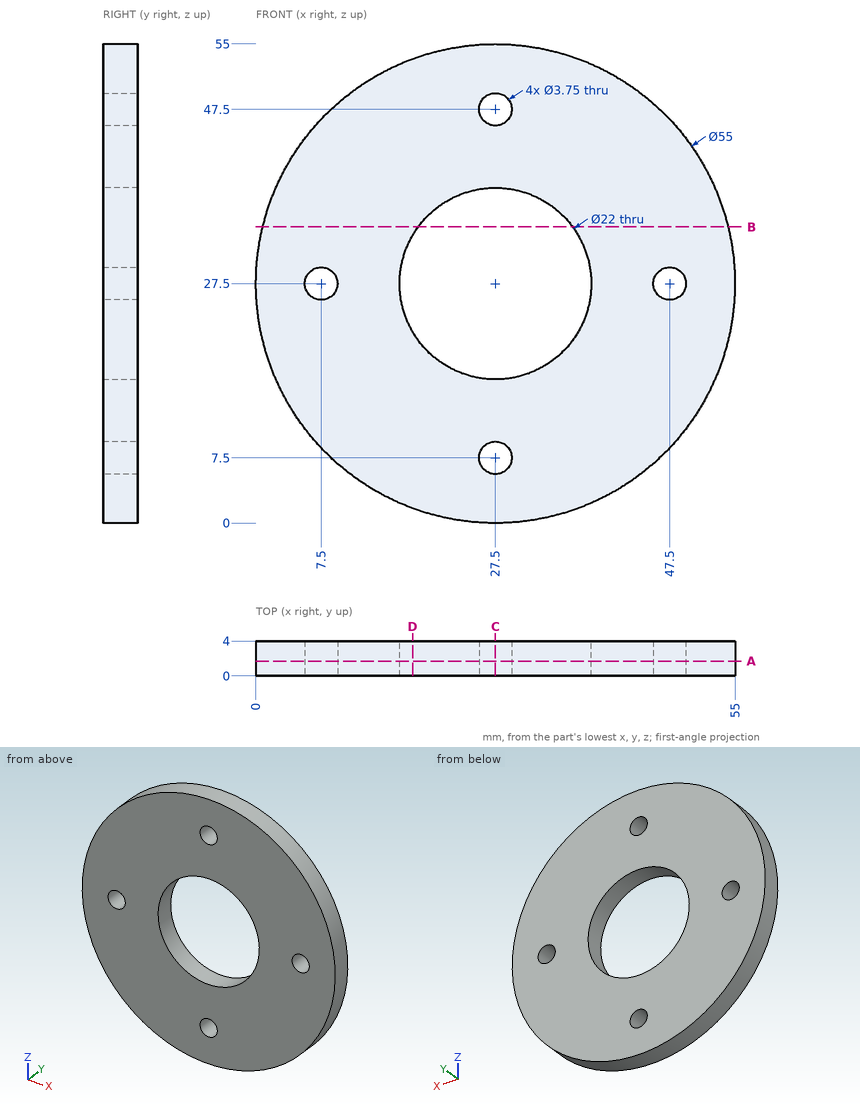
Design review of the part shown in the three views and the two pictorial views. Dimensions are in mm from the part's minimum x, y and z. Give positions to 0.01 mm unless a question says otherwise; leave off trailing zeros. Write each loop counter-clockwise with the first axis right and the second up, starting at its lowest first coordinate (ties: lowest second). Pieces come first, ordered by that corner, then holes. Notation, with made-up numbers: M -18,-11.5 L 20,-11.5 A27 cw 20,19.5 Z; hole C -9.5,40 d1. An arc over 180 degrees is marked long. Answer in a Markdown table with one row per item.
Item 1: For line 1 along X through (y, z) = (2.25, 27.5) (3 decimals); line 2 along X through (y, z) = (0.2, 28.5); line 3 along Z through (x, y) = (28, 1), list the stretches that pass through material, from the lowest coordinate up.
Check sheet entries:
| item | result |
|---|---|
| line 1 | 0 to 5.625, 9.375 to 16.5, 38.5 to 45.625, 49.375 to 55 |
| line 2 | 0.02 to 5.91, 9.09 to 16.55, 38.45 to 45.91, 49.09 to 54.98 |
| line 3 | 0 to 5.69, 9.31 to 16.51, 38.49 to 45.69, 49.31 to 55 |
Item 2: Add section A-A on y = 1.7. Give the boundary of the cut face in (x, z) (3 decimals).
Check sheet entries:
| item | result |
|---|---|
| outline | C 27.5,27.5 d55; hole C 7.5,27.5 d3.75; hole C 27.5,27.5 d22; hole C 27.5,7.5 d3.75; hole C 27.5,47.5 d3.75; hole C 47.5,27.5 d3.75 |
Item 3: Add section D-D on x = 18. Give the boundary of the cut face in (y, z).
Check sheet entries:
| item | result |
|---|---|
| outline | M 0,1.69 L 4,1.69 L 4,21.95 L 0,21.95 Z; M 0,33.05 L 4,33.05 L 4,53.31 L 0,53.31 Z |
Item 4: For P1, Ø1, axis at x = 9.5, y = 3.5, coming from the -Z side; P2, Ø1.5, axis at y = 3, z = 38.5, coming from the -X side; P3, Ø2, axis at y = 2, z = 18.5, coming from the +X side, all flat-tipped, find the tip position at first contact; note any pin that passes through.
Check sheet entries:
| item | result |
|---|---|
| P1 | z = 6.29 |
| P2 | x = 1.98 |
| P3 | x = 53.81 |
Item 5: Add section B-B on z = 34. Give the boundary of the cut face in (x, y), plus the area to 3 significant figures.
Check sheet entries:
| item | result |
|---|---|
| outline | M 0.78,0 L 18.63,0 L 18.63,4 L 0.78,4 Z; M 36.37,0 L 54.22,0 L 54.22,4 L 36.37,4 Z |
| area | 143 mm2 |
Item 6: Add section C-C on x = 27.5. Give the boundary of the cut face in (y, z) (3 decimals).
Check sheet entries:
| item | result |
|---|---|
| outline | M 0,0 L 4,0 L 4,5.625 L 0,5.625 Z; M 0,9.375 L 4,9.375 L 4,16.5 L 0,16.5 Z; M 0,38.5 L 4,38.5 L 4,45.625 L 0,45.625 Z; M 0,49.375 L 4,49.375 L 4,55 L 0,55 Z |
